from build123d import *

# Parameters (mm, degrees)
SKETCH_1_W      = 29.5
SKETCH_1_H      = 13
EXTRUDE_1_DEPTH = 7.2
SKETCH_3_R      = 1.6
EXTRUDE_2_DEPTH = 1.5
EXTRUDE_3_DEPTH = 14.4
SKETCH_5_W      = 10.85
SKETCH_5_H      = 8.4
EXTRUDE_4_DEPTH = 9.9


with BuildPart() as part:
    # 스케치1 → 보스-돌출1 (new body)
    with BuildSketch(Plane.XY):
        Rectangle(SKETCH_1_W, SKETCH_1_H)
    extrude(amount=EXTRUDE_1_DEPTH)

    # 스케치3 → 보스-돌출2 (add)
    # profile 1 of 2: a face of its own
    with BuildSketch(Plane.XY):
        with BuildLine():
            Line((-18.5, 3.75), (-14.75, 3.75))
            Line((-14.75, 3.75), (-14.75, -3.75))
            Line((-14.75, -3.75), (-18.5, -3.75))
            ThreePointArc((-18.5, -3.75), (-22.25, 0), (-18.5, 3.75))
        make_face()
        with Locations((-18.5, 0)):
            Circle(SKETCH_3_R, mode=Mode.SUBTRACT)
    # profile 2 of 2: a face of its own
    with BuildSketch(Plane.XY):
        with BuildLine():
            Line((14.75, -3.75), (14.75, 3.75))
            Line((14.75, 3.75), (18.5, 3.75))
            ThreePointArc((18.5, 3.75), (22.25, 0), (18.5, -3.75))
            Line((18.5, -3.75), (14.75, -3.75))
        make_face()
        with Locations(Location((18.5, 0, 0), (0, 0, 180))):
            Circle(SKETCH_3_R, mode=Mode.SUBTRACT)
    extrude(amount=EXTRUDE_2_DEPTH)

    # 스케치4 → 보스-돌출3 (add)
    with BuildSketch(Plane.XY.offset(7.2)):
        with BuildLine():
            Line((-7.175, -5.95), (-12.625, -5.95))
            ThreePointArc((-12.625, -5.95), (-13.862436867, -5.437436867), (-14.375, -4.2))
            Line((-14.375, -4.2), (-14.375, 4.2))
            ThreePointArc((-14.375, 4.2), (-13.862436867, 5.437436867), (-12.625, 5.95))
            Line((-12.625, 5.95), (-7.175, 5.95))
            ThreePointArc((-7.175, 5.95), (-5.937563133, 5.437436867), (-5.425, 4.2))
            Line((-5.425, 4.2), (-5.425, -4.2))
            ThreePointArc((-5.425, -4.2), (-5.937563133, -5.437436867), (-7.175, -5.95))
        make_face()
        with BuildLine():
            Line((14.375, -4.2), (14.375, 4.2))
            ThreePointArc((14.375, 4.2), (13.862436867, 5.437436867), (12.625, 5.95))
            Line((12.625, 5.95), (7.175, 5.95))
            ThreePointArc((7.175, 5.95), (5.937563133, 5.437436867), (5.425, 4.2))
            Line((5.425, 4.2), (5.425, -4.2))
            ThreePointArc((5.425, -4.2), (5.937563133, -5.437436867), (7.175, -5.95))
            Line((7.175, -5.95), (12.625, -5.95))
            ThreePointArc((12.625, -5.95), (13.862436867, -5.437436867), (14.375, -4.2))
        make_face()
    extrude(amount=EXTRUDE_3_DEPTH)

    # 스케치5 → 보스-돌출4 (add)
    with BuildSketch(Plane.XY.offset(7.2)):
        Rectangle(SKETCH_5_W, SKETCH_5_H)
    extrude(amount=EXTRUDE_4_DEPTH)


solid = part.part
Check sheet for the modelled part. Datum: model origin and axes. Units: mm. A direction names the side the tool comes from. Give positions to 0.01 mm unless a question says otherwise; leave off trailing zeros. Loops run counter-clockwise (first coordinate to the right, second up) from the corner with the lowest first, then second, coordinate; pieces in that order, holes last. Notation, with made-up numbers: M -28.75,86.5 L 23.25,86.5 A13 cw 23.25,109.5 Z; hole C 65.25,66.5 d2. An arc over 180 degrees is marked long. Return JSON: item names as keys, results as strings. Group by question number.
1. Cross-section at D-D on z = 19.75. Record the boundary of the cut face in (x, y) (3 decimals).
2. Tool access check on faces 1 (the flat face through (0, 5, 7.2)), 2 (the cylindrical face through (13.9, 5.4, 14.3)), 3 (the cylindrical face through (-5.9, -5.4, 14.3)), 4 (the flat face through (-10, 5.95, 14)). Record the directions out of +Z, -Z, +X, -X, +Y, -Y that give a thin tool (end or side, any length) a straight path to the whole face; none if there is none.
3. Thickness scan on L1, parallel to Y at x = 18.5, z = 0.5; L2, parallel to Z at x = 17, y = -3.25. Record the ranges inside material, lowest first.
4. Cross-section at A-A on y = 0. Record the boundary of the cut face in (x, z) (3 decimals).
5. Go/stop test with flat-tipped pins: pin 1 (6 mm diameter, centred on y = 2, z = 5, fed in from +X); pin 2 (4 mm diameter, centred on x = -18.5, y = 0, fed in from +Z); pin 3 (1.2 mm diameter, centred on x = 16, z = 1, fed in from -Y). Record where each tip stops, or that it passes through.
6. Cross-section at B-B on z = 14.5. Record the boundary of the cut face in (x, y) (3 decimals), plus the area to 3 significant figures.
7. Mould release check, pull along X, two halves, no side actions. Record for faces 5 (the cylindrical face through (22.25, 0.08, 0.74)), 6 (the flat face through (-14.375, 0, 14)), 7 (the cylindrical face through (-20.1, 0.07, 0.74)): released by +X, released by -X, zero draft, split by the parting line, or undercut.
8. Cross-section at C-C on x = 2. Record the boundary of the cut face in (y, z), plus the area to 3 significant figures.
Return value:
{
 "1": {"outline": "M -14.375,-4.2 A1.75 ccw -12.625,-5.95 L -7.175,-5.95 A1.75 ccw -5.425,-4.2 L -5.425,4.2 A1.75 ccw -7.175,5.95 L -12.625,5.95 A1.75 ccw -14.375,4.2 Z; M 5.425,-4.2 A1.75 ccw 7.175,-5.95 L 12.625,-5.95 A1.75 ccw 14.375,-4.2 L 14.375,4.2 A1.75 ccw 12.625,5.95 L 7.175,5.95 A1.75 ccw 5.425,4.2 Z"},
 "2": {"face 1": "+Z", "face 2": "+Z, +X, +Y", "face 3": "+Z, -Y", "face 4": "+Z, +X, -X, +Y"},
 "3": {"L1": "-3.75 to -1.6, 1.6 to 3.75", "L2": "0 to 1.5"},
 "4": {"outline": "M -22.25,0 L -20.1,0 L -20.1,1.5 L -22.25,1.5 Z; M -16.9,0 L 16.9,0 L 16.9,1.5 L 14.75,1.5 L 14.75,7.2 L 14.375,7.2 L 14.375,21.6 L 5.425,21.6 L 5.425,17.1 L -5.425,17.1 L -5.425,21.6 L -14.375,21.6 L -14.375,7.2 L -14.75,7.2 L -14.75,1.5 L -16.9,1.5 Z; M 20.1,0 L 22.25,0 L 22.25,1.5 L 20.1,1.5 Z"},
 "5": {"pin 1": "x = 14.75", "pin 2": "z = 1.5", "pin 3": "y = -3.75"},
 "6": {"outline": "M -14.375,-4.2 A1.75 ccw -12.625,-5.95 L -7.175,-5.95 A1.75 ccw -5.425,-4.2 L 5.425,-4.2 A1.75 ccw 7.175,-5.95 L 12.625,-5.95 A1.75 ccw 14.375,-4.2 L 14.375,4.2 A1.75 ccw 12.625,5.95 L 7.175,5.95 A1.75 ccw 5.425,4.2 L -5.425,4.2 A1.75 ccw -7.175,5.95 L -12.625,5.95 A1.75 ccw -14.375,4.2 Z", "area": "299 mm^2"},
 "7": {"face 5": "released by +X", "face 6": "released by -X", "face 7": "undercut"},
 "8": {"outline": "M -6.5,0 L 6.5,0 L 6.5,7.2 L 4.2,7.2 L 4.2,17.1 L -4.2,17.1 L -4.2,7.2 L -6.5,7.2 Z", "area": "177 mm^2"}
}
